from build123d import *

# Parameters (mm, degrees)
SKETCH1_W               = 17
SKETCH1_H               = 15
BOSS_EXTRUDE1_DEPTH     = 5
SKETCH2_W               = 3
SKETCH2_H               = 15
SKETCH2_H_2             = 14.97636143
BOSS_EXTRUDE2_DEPTH     = 5
CUT_EXTRUDE2_DEPTH      = 21.185301583
CUT_EXTRUDE2_DEPTH_BACK = 21.185301583
SKETCH4_R               = 1.5
FILLET1_R               = 6
FILLET3_RADIUS          = 1.5
FILLET3_LENGTH          = 14.97636143
FILLET4_RADIUS          = 1.5
FILLET4_LENGTH          = 15
SKETCH5_W               = 17
SKETCH5_H               = 4.2
SKETCH5_W_2             = 16.931812254
CUT_EXTRUDE3_DEPTH      = 14


with BuildPart() as part:
    # Sketch1 → Boss-Extrude1 (new body)
    with BuildSketch(Plane.XY):
        with Locations((-8.5, -7.5)):
            Rectangle(SKETCH1_W, SKETCH1_H)
    extrude(amount=BOSS_EXTRUDE1_DEPTH)

    # Sketch2 → Boss-Extrude2 (add)
    with BuildSketch(Plane.XY.offset(5)):
        with Locations((-6.42, -7.5)):
            Rectangle(SKETCH2_W, SKETCH2_H)
        with Locations((-10.58, -7.511819285)):
            Rectangle(SKETCH2_W, SKETCH2_H_2)
    extrude(amount=BOSS_EXTRUDE2_DEPTH)

    # Sketch4 → Cut-Extrude2 (cut, two sides: drawn at the far end of the back side and taken through both)
    with BuildSketch(Plane(origin=(-9.08, 0, 0), x_dir=(0, 0, -1), z_dir=(1, 0, 0)).offset(-CUT_EXTRUDE2_DEPTH_BACK)):
        with Locations(Location((-7.041389116, -7.762480296, 0), (0, 0, 270))):
            Circle(SKETCH4_R)
    extrude(amount=CUT_EXTRUDE2_DEPTH + CUT_EXTRUDE2_DEPTH_BACK, mode=Mode.SUBTRACT)

    # Fillet1
    # the kernel refuses this fillet: 6 mm, written as the material it takes off along each edge
    with BuildSketch(Plane(origin=(0, -29.754999153, 5), x_dir=(0, 0, -1), z_dir=(0, 1, 0))) as fillet1_piece_1:
        with BuildLine():
            CenterArc((5.901999661, 6), FILLET1_R, 190.369759805, 79.630240195)
            Line((0, 4.92), (0, 0))
            Line((0, 0), (5.901999661, 0))
        make_face()
    extrude(amount=44.509998306, mode=Mode.SUBTRACT)
    # the kernel refuses this fillet: 6 mm, written as the material it takes off along each edge
    with BuildSketch(Plane(origin=(-17, 14.790199458, 5), x_dir=(0, 0, -1), z_dir=(0, -1, 0))) as fillet1_2_piece_1_section:
        with BuildLine():
            CenterArc((6, 5.916079783), FILLET1_R, 180, 80.405931773)
            Line((0, 5.916079783), (0, 0))
            Line((0, 0), (5, 0))
        make_face()
    fillet1_2_piece_1 = extrude(amount=44.580398916, mode=Mode.PRIVATE)
    fillet1_2_piece_1 = split(fillet1_2_piece_1, bisect_by=Plane(origin=(-17, -0.02363857, 5), z_dir=(0, 1, 0)), keep=Keep.TOP, mode=Mode.PRIVATE)
    fillet1_2_piece_1 = split(fillet1_2_piece_1, bisect_by=Plane(origin=(-12.08, 14.790199458, 5), z_dir=(-1, 0, 0)), keep=Keep.TOP, mode=Mode.PRIVATE)
    add(fillet1_2_piece_1, mode=Mode.SUBTRACT)
    with BuildSketch(Plane(origin=(-17, 14.790199458, 5), x_dir=(0, 0, -1), z_dir=(0, -1, 0))) as fillet1_2_piece_2_section:
        with BuildLine():
            CenterArc((6, 5.916079783), FILLET1_R, 180, 80.405931773)
            Line((0, 5.916079783), (0, 0))
            Line((0, 0), (5, 0))
        make_face()
    fillet1_2_piece_2 = extrude(amount=44.580398916, mode=Mode.PRIVATE)
    fillet1_2_piece_2 = split(fillet1_2_piece_2, bisect_by=Plane(origin=(-17, -0.02363857, 5), z_dir=(0, 1, 0)), keep=Keep.TOP, mode=Mode.PRIVATE)
    fillet1_2_piece_2 = split(fillet1_2_piece_2, bisect_by=Plane(origin=(-12.08, 14.790199458, 5), z_dir=(1, 0, 0)), keep=Keep.TOP, mode=Mode.PRIVATE)
    add(fillet1_2_piece_2, mode=Mode.SUBTRACT)
    with BuildSketch(Plane(origin=(-17, 14.790199458, 5), x_dir=(0, 0, -1), z_dir=(0, -1, 0))) as fillet1_2_piece_3_section:
        with BuildLine():
            CenterArc((6, 5.916079783), FILLET1_R, 180, 80.405931773)
            Line((0, 5.916079783), (0, 0))
            Line((0, 0), (5, 0))
        make_face()
    fillet1_2_piece_3 = extrude(amount=44.580398916, mode=Mode.PRIVATE)
    fillet1_2_piece_3 = split(fillet1_2_piece_3, bisect_by=Plane(origin=(-17, -0.02363857, 5), z_dir=(0, -1, 0)), keep=Keep.TOP, mode=Mode.PRIVATE)
    fillet1_2_piece_3 = split(fillet1_2_piece_3, bisect_by=Plane(origin=(-12.08, 14.790199458, 5), z_dir=(-1, 0, 0)), keep=Keep.TOP, mode=Mode.PRIVATE)
    add(fillet1_2_piece_3, mode=Mode.SUBTRACT)

    # Fillet3: full round fillet: the end face becomes a half cylinder, R = half its width
    fillet3_face = Plane((-10.58, -7.511819285, 10), x_dir=(0, -1, 0), z_dir=(0, 0, 1))  # on the end face: x along it, z out of the body
    fillet3_slab = fillet3_face.offset(-FILLET3_RADIUS / 2) * Box(FILLET3_LENGTH, 2 * FILLET3_RADIUS, FILLET3_RADIUS, mode=Mode.PRIVATE)  # the body's end, R deep
    fillet3_round = Plane((-10.58, -7.511819285, 8.5), x_dir=(0, 0, 1), z_dir=(0, -1, 0)) * Cylinder(FILLET3_RADIUS, FILLET3_LENGTH, mode=Mode.PRIVATE)  # its axis R under the face
    add(fillet3_slab - fillet3_round, mode=Mode.SUBTRACT)

    # Fillet4: full round fillet: the end face becomes a half cylinder, R = half its width
    fillet4_face = Plane((-6.42, -7.5, 10), x_dir=(0, -1, 0), z_dir=(0, 0, 1))  # on the end face: x along it, z out of the body
    fillet4_slab = fillet4_face.offset(-FILLET4_RADIUS / 2) * Box(FILLET4_LENGTH, 2 * FILLET4_RADIUS, FILLET4_RADIUS, mode=Mode.PRIVATE)  # the body's end, R deep
    fillet4_round = Plane((-6.42, -7.5, 8.5), x_dir=(0, 0, 1), z_dir=(0, -1, 0)) * Cylinder(FILLET4_RADIUS, FILLET4_LENGTH, mode=Mode.PRIVATE)  # its axis R under the face
    add(fillet4_slab - fillet4_round, mode=Mode.SUBTRACT)

    # Sketch5 → Cut-Extrude3 (cut)
    with BuildSketch(Plane.XY):
        with Locations((-8.5, -2.1)):
            Rectangle(SKETCH5_W, SKETCH5_H)
        with Locations((-8.534093873, -12.9)):
            Rectangle(SKETCH5_W_2, SKETCH5_H)
    extrude(amount=CUT_EXTRUDE3_DEPTH, mode=Mode.SUBTRACT)


solid = part.part
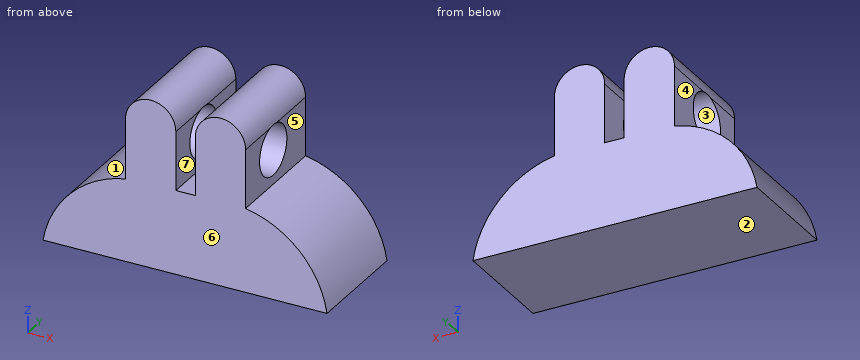
Input: part model. Units: mm. Frame: model coordinates. Face numbers are marked on the shaded views. A direction names the side the tool comes from. Round coordinates to 2 decimals unless told otherwise and drop trailing zeros. Order: outer loops, then holes, each group sorted by start corner. A loop starts at its lowest first (then second) coordinate and runs counter-clockwise, first axis right, second up. Notation, with made-up numbers: (20.25, 9) - (60.25, 9) arc R34 ccw to (60.25, 44) - close; hole circle Ø1 at (36.25, 66). An arc over 180 degrees is marked (long way). Answer as a JSON object with one key per item and string values. Group by question number.
(1) Cut plane B-B (z = 9.75). Return loops of the section in (x, y).
(2) Pin query (flat end, axial travel): P1, Ø3, axis at y = -6.5, z = 6.5, coming from the -X side; P2, Ø1.1, axis at y = -8.5, z = 6, coming from the +X side; P3, Ø2, axis at x = -3, z = 5, coming from the -Y side. Return the tip coordinate at first contact, or that it passes through.
(3) Reachability of the marked faces 4, 5, 6 and 7 from +Z, -Z, +X, -X, +Y, -Y: full face, straight path, thin tool, end or side. Return the list, or none.
(4) Draft query along Z for the marked faces 1, 2 and 3. Return one class per face: released by +Z, released by -Z, zero draft, split by the parting line, or undercut.
(5) Material intervals for probe 1 along X at (y, z) = (-5.5, 8.5); probe 2 along Y at (x, z) = (-5.5, 7.75); probe 3 along Z at (x, y) = (-5.75, -7.5), sorted ascending. Write a range as from..to.
(6) Cut plane C-C (z = 8). Return loops of the section in (x, y), then the cut area to 3 significant figures.
(7) Cut plane A-A (y = -7). Return loops of the section in (x, z).
(8) Cut plane D-D (y = -4.75). Return loops of the section in (x, z).
Here are the results:
{
 "1": {"outline": "(-11.41, -10.8) - (-9.75, -10.8) - (-9.75, -4.2) - (-11.41, -4.2) - close; (-7.25, -10.8) - (-5.59, -10.8) - (-5.59, -4.2) - (-7.25, -4.2) - close"},
 "2": {"P1": "stops at x = -12.08", "P2": "stops at x = -4.92", "P3": "stops at y = -10.8"},
 "3": {"face 4": "+Z, -X, +Y, -Y", "face 5": "+Z, +X, +Y, -Y", "face 6": "+Z, -Z, +X, -X, -Y", "face 7": "+Z, +Y, -Y"},
 "4": {"face 1": "released by +Z", "face 2": "released by -Z", "face 3": "undercut"},
 "5": {"probe 1": "x = -12.08..-9.08, -7.92..-4.92", "probe 2": "y = -10.8..-9.08, -6.44..-4.2", "probe 3": "z = 0..5.56, 8.52..9.84"},
 "6": {"outline": "(-12.08, -10.8) - (-9.08, -10.8) - (-9.08, -8.92) - (-12.08, -8.92) - close; (-12.08, -6.61) - (-9.08, -6.61) - (-9.08, -4.2) - (-12.08, -4.2) - close; (-7.92, -10.8) - (-4.92, -10.8) - (-4.92, -8.92) - (-7.92, -8.92) - close; (-7.92, -6.61) - (-4.92, -6.61) - (-4.92, -4.2) - (-7.92, -4.2) - close", "area": "25.8 mm^2"},
 "7": {"outline": "(-17, 0) - (-0.07, 0) arc R6 ccw to (-4.92, 5) - (-4.92, 5.75) - (-7.92, 5.75) - (-7.92, 5) - (-9.08, 5) - (-9.08, 5.75) - (-12.08, 5.75) - (-12.08, 4.92) arc R6 ccw to start; (-12.08, 8.33) - (-9.08, 8.33) - (-9.08, 8.5) arc R1.5 ccw to (-12.08, 8.5) - close; (-7.92, 8.33) - (-4.92, 8.33) - (-4.92, 8.5) arc R1.5 ccw to (-7.92, 8.5) - close"},
 "8": {"outline": "(-17, 0) - (-0.07, 0) arc R6 ccw to (-4.92, 5) - (-4.92, 8.5) arc R1.5 ccw to (-7.92, 8.5) - (-7.92, 5) - (-9.08, 5) - (-9.08, 8.5) arc R1.5 ccw to (-12.08, 8.5) - (-12.08, 4.92) arc R6 ccw to start"}
}
